Geometry: final body of the model. Coordinates: model frame, mm. A direction names the side the tool comes from. Give positions to 0.01 mm unless a question says otherwise; leave off trailing zeros. Order: outer loops, then holes, each group sorted by start corner. A loop starts at its lowest first (then second) coordinate and runs counter-clockwise, first axis right, second up. Notation, with made-up numbers: (23.5, 87) - (50.5, 87) arc R16 cw to (50.5, 110) - close; hole circle Ø2 at (-22.75, 77.5). An arc over 180 degrees is marked (long way). Use one line per item in the form item = value.
from build123d import *

# Parameters (mm, degrees)
SKETCH1_W           = 97
SKETCH1_H           = 29.491999944
BOSS_EXTRUDE1_DEPTH = 160.778000008
SKETCH2_W           = 95.4125
SKETCH2_H           = 6.35
CUT_EXTRUDE1_DEPTH  = 12.7
CUT_EXTRUDE2_DEPTH  = 19.967
SKETCH4_R           = 3.175
SKETCH4_R_2         = 0.79375
CUT_EXTRUDE3_DEPTH  = 6.35
FILLET1_R           = 0.79375
CUT_EXTRUDE4_DEPTH  = 1.27
SKETCH6_W           = 10.16
SKETCH6_H           = 27.904499944
CUT_EXTRUDE6_DEPTH  = 4.445
SKETCH7_R           = 1.5
CUT_EXTRUDE7_DEPTH  = 6.35
SKETCH8_R           = 1
SKETCH8_R_2         = 1.75
CUT_EXTRUDE8_DEPTH  = 6.35
CUT_EXTRUDE9_DEPTH  = 95.4125


with BuildPart() as part:
    # Sketch1 → Boss-Extrude1 (new body)
    with BuildSketch(Plane.XY):
        with Locations((48.5, 14.745999972)):
            Rectangle(SKETCH1_W, SKETCH1_H)
    extrude(amount=-BOSS_EXTRUDE1_DEPTH)

    # Sketch2 → Cut-Extrude1 (cut)
    with BuildSketch(Plane.XY):
        Polygon((95.4125, 9.525), (95.4125, 29.491999944), (0, 29.491999944), (0, 9.525), (10.16, 9.525), (10.16, 19.966999944), (11.557, 19.966999944), (11.557, 14.2875), (19.685, 14.2875), (19.685, 19.966999944), (21.082, 19.966999944), (21.082, 14.2875), (29.21, 14.2875), (29.21, 19.966999944), (30.607, 19.966999944), (30.607, 14.2875), (38.735, 14.2875), (38.735, 19.966999944), (40.132, 19.966999944), (40.132, 14.2875), (48.26, 14.2875), (48.26, 19.966999944), (49.657, 19.966999944), (49.657, 14.2875), (57.785, 14.2875), (57.785, 19.966999944), (59.182, 19.966999944), (59.182, 14.2875), (67.31, 14.2875), (67.31, 19.966999944), (68.707, 19.966999944), (68.707, 14.2875), (76.835, 14.2875), (76.835, 19.966999944), (78.232, 19.966999944), (78.232, 9.525), (83.64725, 9.525), (83.64725, 17.145), (89.99725, 17.145), (89.99725, 9.525), align=None)
        with Locations((47.70625, 4.7625)):
            Rectangle(SKETCH2_W, SKETCH2_H)
    extrude(amount=-CUT_EXTRUDE1_DEPTH, mode=Mode.SUBTRACT)

    # Sketch3 → Cut-Extrude2 (cut)
    with BuildSketch(Plane(origin=(0, 29.491999944, 0), x_dir=(1, 0, 0), z_dir=(0, 1, 0))):
        with BuildLine():
            ThreePointArc((89.99725, 6.35), (86.82225, 3.175), (83.64725, 6.35))
            Line((83.64725, 6.35), (83.64725, 0))
            Line((83.64725, 0), (89.99725, 0))
            Line((89.99725, 0), (89.99725, 6.35))
        make_face()
        with BuildLine():
            Line((89.99725, 12.7), (83.64725, 12.7))
            Line((83.64725, 12.7), (83.64725, 6.35))
            ThreePointArc((83.64725, 6.35), (86.82225, 9.525), (89.99725, 6.35))
            Line((89.99725, 6.35), (89.99725, 12.7))
        make_face()
    extrude(amount=-CUT_EXTRUDE2_DEPTH, mode=Mode.SUBTRACT)

    # Sketch4 → Cut-Extrude3 (cut)
    with BuildSketch(Plane(origin=(0, 9.525, 0), x_dir=(1, 0, 0), z_dir=(0, 1, 0))):
        with Locations((86.82225, 6.35)):
            Circle(SKETCH4_R)
        with Locations((86.82225, 6.35)):
            Circle(SKETCH4_R_2, mode=Mode.SUBTRACT)
    extrude(amount=CUT_EXTRUDE3_DEPTH, mode=Mode.SUBTRACT)

    # Fillet1
    fillet1_edges = [part.edges().sort_by_distance(p)[0] for p in [
        (83.64725, 17.145, -6.35),
    ]]
    fillet(fillet1_edges, radius=FILLET1_R)

    # Sketch5 → Cut-Extrude4 (cut)
    with BuildSketch(Plane(origin=(0, 17.145, 0), x_dir=(1, 0, 0), z_dir=(0, 1, 0))):
        Polygon((86.44125, 8.73125), (86.44125, 6.731), (84.441, 6.731), (84.441, 5.969), (86.44125, 5.969), (86.44125, 3.96875), (87.20325, 3.96875), (87.20325, 5.969), (89.2035, 5.969), (89.2035, 6.731), (87.20325, 6.731), (87.20325, 8.73125), align=None)
    extrude(amount=-CUT_EXTRUDE4_DEPTH, mode=Mode.SUBTRACT)

    # Sketch6 → Cut-Extrude6 (cut)
    with BuildSketch(Plane(origin=(0, 0, -160.778000008), x_dir=(-1, 0, 0), z_dir=(0, 0, -1))):
        with Locations((-90.3325, 15.539749972)):
            Rectangle(SKETCH6_W, SKETCH6_H)
    extrude(amount=-CUT_EXTRUDE6_DEPTH, mode=Mode.SUBTRACT)

    # Sketch7 → Cut-Extrude7 (cut)
    with BuildSketch(Plane(origin=(97, 0, 0), x_dir=(0, 0, -1), z_dir=(1, 0, 0))):
        with Locations((6.5024, 26.289)):
            Circle(SKETCH7_R)
        with Locations((22.225, 15.24)):
            Circle(SKETCH7_R)
        with Locations((138.684, 6)):
            Circle(SKETCH7_R)
        with Locations((138.684, 23.9832)):
            Circle(SKETCH7_R)
        with BuildLine():
            Line((160.778000008, 15.974), (156.3624, 15.974))
            ThreePointArc((156.3624, 15.974), (154.6124, 14.224), (156.3624, 12.474))
            Line((156.3624, 12.474), (160.778000008, 12.474))
            Line((160.778000008, 12.474), (160.778000008, 15.974))
        make_face()
    extrude(amount=-CUT_EXTRUDE7_DEPTH, mode=Mode.SUBTRACT)

    # Sketch8 → Cut-Extrude8 (cut)
    with BuildSketch(Plane.XZ):
        with Locations((65.25, -24.003)):
            Circle(SKETCH8_R)
        with Locations((65.25, -102.87)):
            Circle(SKETCH8_R)
        with Locations((5.461, -4.4958)):
            Circle(SKETCH8_R_2)
        with BuildLine():
            Line((92.146, -160.778000008), (92.146, -157.988))
            ThreePointArc((92.146, -157.988), (90.396, -156.238), (88.646, -157.988))
            Line((88.646, -157.988), (88.646, -160.778000008))
            Line((88.646, -160.778000008), (92.146, -160.778000008))
        make_face()
    extrude(amount=-CUT_EXTRUDE8_DEPTH, mode=Mode.SUBTRACT)

    # Sketch9 → Cut-Extrude9 (cut)
    with BuildSketch(Plane.ZY):
        Polygon((-160.778000008, 7.874), (-156.333000008, 12.319), (-156.333000008, 29.491999944), (-160.778000008, 29.491999944), align=None)
    extrude(amount=-CUT_EXTRUDE9_DEPTH, mode=Mode.SUBTRACT)


solid = part.part
(1) Ray query, line 1 along Z through (x, y) = (65.25, 5); line 2 along Z through (x, y) = (86, 27.5); line 3 along Y through (x, z) = (63.5, -12). Return the intervals inside material, ascending.
Computed values:
line_1 = -160.78 to -103.87, -101.87 to -25, -23 to -12.7
line_2 = -156.33 to -12.7
line_3 = 0 to 1.59, 7.94 to 14.29
(2) Contact query for flat-ended pins moving along their axis: pin 1 Ø10 at (x, z) = (70.5, -3.5) entering from +Y; pin 2 Ø6 at (y, z) = (15.5, -9) entering from -X; pin 3 Ø4 at (x, z) = (36, -8.5) entering from +Y. Output: stop coordinate, or through.
Computed values:
pin_1 = 19.97
pin_2 = 10.16
pin_3 = 14.29
(3) Cut plane A-A on x = 13.5. Output: boundary loops of the cut face in (y, z), plus the area to 3 significant figures.
Computed values:
outline = (0, -160.78) - (7.87, -160.78) - (12.32, -156.33) - (29.49, -156.33) - (29.49, -12.7) - (14.29, -12.7) - (14.29, 0) - (7.94, 0) - (7.94, -12.7) - (1.59, -12.7) - (1.59, 0) - (0, 0) - close
area = 4,380 mm²
(4) Reachability of faces 5 (the face through (87, 1.587, -159)), 6 (the face through (84.3, 16.12, -8.28)), 7 (the face through (59.182, 17, -6)) from +Z, -Z, +X, -X, +Y, -Y: full face, straight path, thin tool, end or side. Return the list, or none.
Computed values:
face_5 = -Z, +Y
face_6 = +Y
face_7 = +Z, +Y
(5) Pull-direction query (Y, two-part tool) for faces 1 (the face through (97, 15, -79)), 2 (the face through (87.5, 15.875, -7.1)), 3 (the face through (42.029, 10.065, -158.587)), 4 (the face through (93.869, 15.306, -20.726)); classes: released by +Y, released by -Y, zero draft, split by the parting line, or undercut.
Computed values:
face_1 = zero draft
face_2 = undercut
face_3 = released by +Y
face_4 = undercut
